Work out the finished part from the listing and answer in its coordinate system (mm). Give positions to 0.01 mm unless a question says otherwise; leave off trailing zeros. Write each loop counter-clockwise with the first axis right and the second up, starting at its lowest first coordinate (ties: lowest second). Pieces come first, ordered by that corner, then holes. Notation, with made-up numbers: (-3, 38) -> (56, 38) arc R20 ccw to (56, 77) -> close; hole circle Ø7 at (40, 79). An arc over 180 degrees is marked (long way). Use a Markdown table: item, result. Add a question column.
Q1. Each of these flat-tipped pins is pushed along its axis until it touches: pin 1 Ø2.5 at (x, y) = (30, 85) entering from -Z; pin 2 Ø6.5 at (x, y) = (170, 15) entering from +Z. Where does it stop, or does it pass through?
Q2. Consider line 1 (Y direction, x = 30, z = 6.25). Determine where the line is inside the solid, lowest interval first.
Q3. Section A-A, the plane x = 70 is taken. Give the vertices of the cut face in (y, z), plus the area to 3 significant figures.
Q4. Section B-B, the plane y = 85 is taken. Give the vertices of the cut face in (x, z), plus the area to 3 significant figures.
from build123d import *

# Parameters (mm, degrees)
SKETCH_W  = 200
SKETCH_H  = 100
SKETCH_R  = 2
PAD_DEPTH = 10
FILLET_R  = 3


with BuildPart() as part:
    # Sketch → Pad (new body)
    with BuildSketch(Plane.XY):
        with Locations((100, 50)):
            Rectangle(SKETCH_W, SKETCH_H)
        with Locations((30, 85)):
            Circle(SKETCH_R, mode=Mode.SUBTRACT)
        with Locations((30, 15)):
            Circle(SKETCH_R, mode=Mode.SUBTRACT)
        with Locations((170, 85)):
            Circle(SKETCH_R, mode=Mode.SUBTRACT)
        with Locations((170, 15)):
            Circle(SKETCH_R, mode=Mode.SUBTRACT)
        with Locations((50, 85)):
            Circle(SKETCH_R, mode=Mode.SUBTRACT)
        with Locations((50, 15)):
            Circle(SKETCH_R, mode=Mode.SUBTRACT)
        with Locations((150, 85)):
            Circle(SKETCH_R, mode=Mode.SUBTRACT)
        with Locations((150, 15)):
            Circle(SKETCH_R, mode=Mode.SUBTRACT)
        with Locations((70, 85)):
            Circle(SKETCH_R, mode=Mode.SUBTRACT)
        with Locations((70, 15)):
            Circle(SKETCH_R, mode=Mode.SUBTRACT)
        with Locations((130, 15)):
            Circle(SKETCH_R, mode=Mode.SUBTRACT)
        with Locations((130, 85)):
            Circle(SKETCH_R, mode=Mode.SUBTRACT)
    extrude(amount=PAD_DEPTH)

    # Fillet
    fillet_edges = [part.edges().sort_by_distance(p)[0] for p in [
        (200, 0, 5),
        (0, 0, 5),
        (200, 100, 5),
        (0, 100, 5),
    ]]
    fillet(fillet_edges, radius=FILLET_R)


solid = part.part
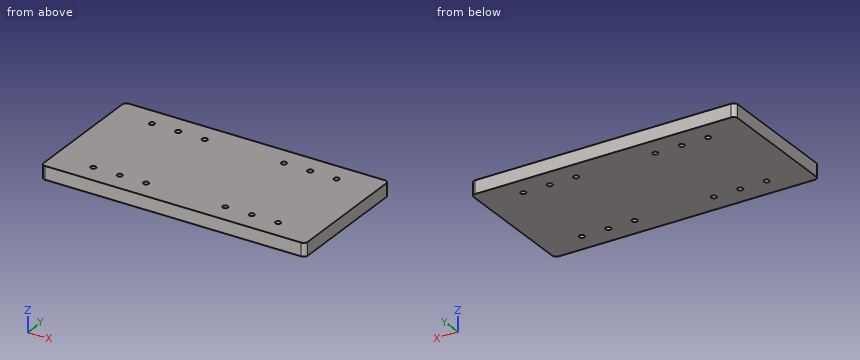
Result set:
| question | item | result |
|---|---|---|
| 1 | pin 1 | passes through |
| 1 | pin 2 | stops at z = 10 |
| 2 | line 1 | y = 0 to 13, 17 to 83, 87 to 100 |
| 3 | outline | (0, 0) -> (13, 0) -> (13, 10) -> (0, 10) -> close; (17, 0) -> (83, 0) -> (83, 10) -> (17, 10) -> close; (87, 0) -> (100, 0) -> (100, 10) -> (87, 10) -> close |
| 3 | area | 920 mm2 |
| 4 | outline | (0, 0) -> (28, 0) -> (28, 10) -> (0, 10) -> close; (32, 0) -> (48, 0) -> (48, 10) -> (32, 10) -> close; (52, 0) -> (68, 0) -> (68, 10) -> (52, 10) -> close; (72, 0) -> (128, 0) -> (128, 10) -> (72, 10) -> close; (132, 0) -> (148, 0) -> (148, 10) -> (132, 10) -> close; (152, 0) -> (168, 0) -> (168, 10) -> (152, 10) -> close; (172, 0) -> (200, 0) -> (200, 10) -> (172, 10) -> close |
| 4 | area | 1,760 mm2 |
